The listing builds one solid part. Answer for the finished solid, in the listing's coordinates (mm). Face numbers are marked on the shaded views. A direction names the side the tool comes from. Round coordinates to 2 decimals unless told otherwise and drop trailing zeros. Loops run counter-clockwise (first coordinate to the right, second up) from the corner with the lowest first, then second, coordinate; pieces in that order, holes last. Notation, with made-up numbers: M -23,36.5 L 6,36.5 A5 cw 6,43.5 Z; hole C 2.25,-3 d1. An arc over 180 degrees is marked long. Put each result on its own line as item: value. Start each with the question number.
(1) Section C-C, the plane y = -9.25 is taken. Determine the outline of the cut face in (x, z), then the cut area to 3 significant figures.
(2) Which of the six approach directions +Z, -Z, +X, -X, +Y, -Y give full straight-line access (tool end or side, diameter ignored) to the marked faces 1 and 2?
(3) Section A-A, the plane z = 1.25 is taken. Determine the outline of the cut face in (x, y).
(4) Straight lines are drawn through the part: line 1 (Y direction, x = -1, z = 3.75); line 2 (X direction, y = -6, z = -0.75); line 3 (X direction, y = 1.25, z = -2.25). For each, find the intervals that lie inside material, in ascending order.
(5) Flat-ended cylindrical pins translate along their axes: P1, Ø5, axis at y = -5.5, z = -1, coming from the -X side; P2, Ø3, axis at x = -3, z = 3.5, coming from the -Y side; P3, Ø3, axis at x = 3, y = -4.5, coming from the -Z side. Find the tip coordinate at first contact, or state that the pin passes through.
(6) Section D-D, the plane x = -3 is taken. Determine the outline of the cut face in (y, z), then the cut area to 3 significant figures.
(7) Section B-B, the plane x = 0 is taken. Determine the outline of the cut face in (y, z).
```python
from build123d import *

# Parameters (mm, degrees)
SKETCH1_R                = 5
SKETCH1_R_2              = 2.5
BOSS_EXTRUDE2_DEPTH      = 3
BOSS_EXTRUDE3_DEPTH      = 10.885792211
BOSS_EXTRUDE3_DEPTH_BACK = 3
SKETCH5_R                = 2.5
CUT_EXTRUDE3_START       = -0.2
SKETCH6_R                = 5
CUT_EXTRUDE3_DEPTH       = 0.2


with BuildPart() as part:
    # Sketch1 → Boss-Extrude2 (new body)
    with BuildSketch(Plane(origin=(0, 0, 0), x_dir=(1, 0, 0), z_dir=(0, 1, 0))):
        with Locations(Location((0, 0, 0), (0, 0, 270))):
            Circle(SKETCH1_R)
        with Locations(Location((0, 0, 0), (0, 0, 270))):
            Circle(SKETCH1_R_2, mode=Mode.SUBTRACT)
    extrude(amount=BOSS_EXTRUDE2_DEPTH)

    # Sketch5 → Boss-Extrude3 (add, two sides: drawn at the far end of the back side and taken through both)
    with BuildSketch(Plane.XZ.offset(-BOSS_EXTRUDE3_DEPTH_BACK)):
        with Locations(Location((0, 0, 0), (0, 0, 270))):
            Circle(SKETCH5_R)
    extrude(amount=BOSS_EXTRUDE3_DEPTH + BOSS_EXTRUDE3_DEPTH_BACK)

    # Sketch6 → Cut-Extrude3 (cut)
    with BuildSketch(Plane(origin=(0, 3, 0), x_dir=(1, 0, 0), z_dir=(0, 1, 0)).offset(CUT_EXTRUDE3_START)):
        with Locations(Location((0, 0, 0), (0, 0, 270))):
            Circle(SKETCH6_R)
    extrude(amount=CUT_EXTRUDE3_DEPTH, mode=Mode.SUBTRACT)


solid = part.part
```
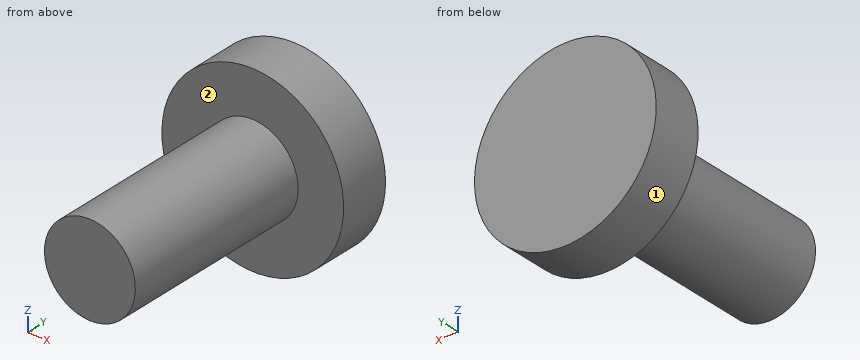
Recorded:
1. outline: C 0,0 d5
1. area: 19.6 mm²
2. face 1: +Y, -Y
2. face 2: -Y
3. outline: M -4.84,0 L -2.17,0 L -2.17,-10.89 L 2.17,-10.89 L 2.17,0 L 4.84,0 L 4.84,2.8 L -4.84,2.8 Z
4. line 1: y = 0 to 2.8
4. line 2: x = -2.38 to 2.38
4. line 3: x = -4.47 to 4.47
5. P1: stops at x = -2.5
5. P2: stops at y = 0
5. P3: stops at z = -2
6. outline: M 0,-4 L 2.8,-4 L 2.8,4 L 0,4 Z
6. area: 22.4 mm²
7. outline: M -10.89,-2.5 L 0,-2.5 L 0,-5 L 2.8,-5 L 2.8,5 L 0,5 L 0,2.5 L -10.89,2.5 Z
